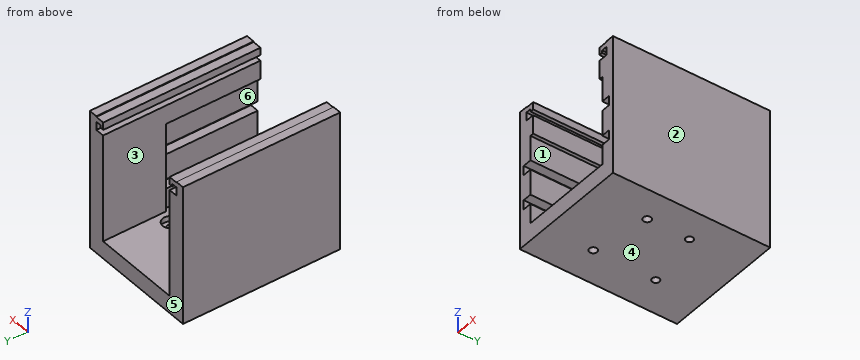
```python
from build123d import *

# Parameters (mm, degrees)
SKETCH1_W                                     = 90
SKETCH1_H                                     = 70
BOSS_EXTRUDE1_DEPTH                           = 10
SKETCH2_W                                     = 8
SKETCH2_H                                     = 90
BOSS_EXTRUDE2_DEPTH                           = 51
SKETCH3_W                                     = 5.1
SKETCH3_H                                     = 5.4
CUT_EXTRUDE1_DEPTH                            = 54
SKETCH14_W                                    = 10
SKETCH14_H                                    = 90
BOSS_EXTRUDE6_DEPTH                           = 11.75
SKETCH15_W                                    = 4.9
SKETCH15_H                                    = 90
BOSS_EXTRUDE7_DEPTH                           = 7
SKETCH17_W                                    = 90
SKETCH17_H                                    = 2.8
BOSS_EXTRUDE8_DEPTH                           = 5
SKETCH16_W                                    = 5.1
SKETCH16_H                                    = 90
CUT_EXTRUDE3_DEPTH                            = 1
BOSS_EXTRUDE9_START                           = -1.5
SKETCH18_W                                    = 2
SKETCH18_H                                    = 90
BOSS_EXTRUDE9_DEPTH                           = 4.3
SKETCH43_W                                    = 36
SKETCH43_H                                    = 51
BOSS_EXTRUDE10_DEPTH                          = 2
SKETCH21_R                                    = 2.1
CUT_EXTRUDE7_DEPTH                            = 99.030926243
CBORE_FOR_M4_PAN_HEAD_MACHINE_SCREW4_AT_COUNT = 2
CBORE_FOR_M4_PAN_HEAD_MACHINE_SCREW4_AT_PITCH = 33.407334524
ADVANCEDHOLE1_START                           = 6.9
ADVANCEDHOLE1_OUTLINE_R                       = 4.5
ADVANCEDHOLE1_OUTLINE_R_2                     = 2.1
ADVANCEDHOLE1_DEPTH                           = 3.1


# Read off the part's stored shape, not the designer's step: AdvancedHole1
with BuildPart() as part:
    # Sketch1 → Boss-Extrude1 (new body)
    with BuildSketch(Plane(origin=(0, 0, 0), x_dir=(0, 1, 0), z_dir=(0, 0, 1))):
        Rectangle(SKETCH1_W, SKETCH1_H)
    extrude(amount=BOSS_EXTRUDE1_DEPTH)

    # Sketch2 → Boss-Extrude2 (add)
    with BuildSketch(Plane.XY.offset(10)):
        with Locations((-31, 0)):
            Rectangle(SKETCH2_W, SKETCH2_H)
        with Locations((31, 0)):
            Rectangle(SKETCH2_W, SKETCH2_H)
    extrude(amount=BOSS_EXTRUDE2_DEPTH)

    # Sketch3 → Cut-Extrude1 (cut)
    with BuildSketch(Plane.XZ.offset(45)):
        with Locations((-29.55, 24)):
            Rectangle(SKETCH3_W, SKETCH3_H)
        with Locations((-29.55, 44)):
            Rectangle(SKETCH3_W, SKETCH3_H)
        with Locations((29.55, 24)):
            Rectangle(SKETCH3_W, SKETCH3_H)
        with Locations((29.55, 44)):
            Rectangle(SKETCH3_W, SKETCH3_H)
    extrude(amount=-CUT_EXTRUDE1_DEPTH, mode=Mode.SUBTRACT)

    # Sketch14 → Boss-Extrude6 (add)
    with BuildSketch(Plane.XY.offset(61)):
        with Locations((30, 0)):
            Rectangle(SKETCH14_W, SKETCH14_H)
    boss_extrude6 = extrude(amount=BOSS_EXTRUDE6_DEPTH)

    # Sketch15 → Boss-Extrude7 (add)
    with BuildSketch(Plane.XY.offset(72.75)):
        with Locations((32.55, 0)):
            Rectangle(SKETCH15_W, SKETCH15_H)
    boss_extrude7 = extrude(amount=BOSS_EXTRUDE7_DEPTH)

    # Sketch17 → Boss-Extrude8 (add)
    with BuildSketch(Plane(origin=(30.1, 0, 0), x_dir=(0, -1, 0), z_dir=(-1, 0, 0))):
        with Locations((0, 77.95)):
            Rectangle(SKETCH17_W, SKETCH17_H)
    boss_extrude8 = extrude(amount=BOSS_EXTRUDE8_DEPTH)

    # Sketch16 → Cut-Extrude3 (cut)
    with BuildSketch(Plane.XY.offset(72.75)):
        with Locations((27.55, 0)):
            Rectangle(SKETCH16_W, SKETCH16_H)
    cut_extrude3 = extrude(amount=-CUT_EXTRUDE3_DEPTH, mode=Mode.SUBTRACT)

    # Sketch18 → Boss-Extrude9 (add)
    with BuildSketch(Plane.XY.offset(76.55).offset(BOSS_EXTRUDE9_START)):
        with Locations((25.9, 0)):
            Rectangle(SKETCH18_W, SKETCH18_H)
    boss_extrude9 = extrude(amount=BOSS_EXTRUDE9_DEPTH)

    # Sketch43 → Boss-Extrude10 (add)
    with BuildSketch(Plane(origin=(27, 0, 0), x_dir=(0, -1, 0), z_dir=(-1, 0, 0))):
        with Locations((-27, 35.5)):
            Rectangle(SKETCH43_W, SKETCH43_H)
    boss_extrude10 = extrude(amount=BOSS_EXTRUDE10_DEPTH)

    # Mirror2: Boss-Extrude6, Boss-Extrude7, Boss-Extrude8, Cut-Extrude3, Boss-Extrude9, Boss-Extrude10 across plane
    add(boss_extrude6.mirror(Plane(origin=(0, 0, 0), x_dir=(0, 0, 1), z_dir=(1, 0, 0))))
    add(boss_extrude7.mirror(Plane(origin=(0, 0, 0), x_dir=(0, 0, 1), z_dir=(1, 0, 0))))
    add(boss_extrude8.mirror(Plane(origin=(0, 0, 0), x_dir=(0, 0, 1), z_dir=(1, 0, 0))))
    add(cut_extrude3.mirror(Plane(origin=(0, 0, 0), x_dir=(0, 0, 1), z_dir=(1, 0, 0))), mode=Mode.SUBTRACT)
    add(boss_extrude9.mirror(Plane(origin=(0, 0, 0), x_dir=(0, 0, 1), z_dir=(1, 0, 0))))
    add(boss_extrude10.mirror(Plane(origin=(0, 0, 0), x_dir=(0, 0, 1), z_dir=(1, 0, 0))))

    # Sketch21 → Cut-Extrude7 (cut, through all)
    with BuildSketch(Plane(origin=(0, 0, 0), x_dir=(1, 0, 0), z_dir=(0, 0, -1))):
        with Locations((17.5, 12.1)):
            Circle(SKETCH21_R)
        with Locations(Location((17.5, -12.1, 0), (0, 0, 180))):
            Circle(SKETCH21_R)
        with Locations(Location((-15.4, -17.9, 0), (0, 0, 180))):
            Circle(SKETCH21_R)
        with Locations((-15.4, 17.9)):
            Circle(SKETCH21_R)
    extrude(amount=-CUT_EXTRUDE7_DEPTH, mode=Mode.SUBTRACT)

    # Sketch30 → CBORE for M4 Pan Head Machine Screw4 (revolve, cut)
    with BuildSketch(Plane(origin=(17.5, -12.1, 10), x_dir=(0, -1, 0), z_dir=(1, 0, 0))):
        Polygon((0, 0), (0, 10), (2.25, 10), (2.25, 3.1), (4.5, 3.1), (4.5, 0.025), (4.525, 0), align=None)
    cbore_for_m4_pan_head_machine_screw4 = revolve(axis=Axis((17.5, -12.1, 16.35), (0, 0, -1)), mode=Mode.SUBTRACT)

    # CBORE for M4 Pan Head Machine Screw4 at: CBORE for M4 Pan Head Machine Screw4 ×2
    with Locations(*[Vector(-0.9848136784555953, -0.1736145694541778, 0) * (i * CBORE_FOR_M4_PAN_HEAD_MACHINE_SCREW4_AT_PITCH) for i in range(1, CBORE_FOR_M4_PAN_HEAD_MACHINE_SCREW4_AT_COUNT)]):
        add(cbore_for_m4_pan_head_machine_screw4, mode=Mode.SUBTRACT)

    # AdvancedHole1 outline → AdvancedHole1 (cut)
    # profile 1 of 2: a face of its own
    with BuildSketch(Plane.XY.offset(ADVANCEDHOLE1_START)):
        with Locations((17.5, 12.1)):
            Circle(ADVANCEDHOLE1_OUTLINE_R)
        with Locations((17.5, 12.1)):
            Circle(ADVANCEDHOLE1_OUTLINE_R_2, mode=Mode.SUBTRACT)
    # profile 2 of 2: a face of its own
    with BuildSketch(Plane.XY.offset(ADVANCEDHOLE1_START)):
        with Locations((-15.4, 17.9)):
            Circle(ADVANCEDHOLE1_OUTLINE_R)
        with Locations((-15.4, 17.9)):
            Circle(ADVANCEDHOLE1_OUTLINE_R_2, mode=Mode.SUBTRACT)
    extrude(amount=ADVANCEDHOLE1_DEPTH, mode=Mode.SUBTRACT)


solid = part.part
```
The listing builds one solid part. Answer for the finished solid, in the listing's coordinates (mm). Face numbers are marked on the shaded views. A direction names the side the tool comes from. Round coordinates to 2 decimals unless told otherwise and drop trailing zeros. Loops run counter-clockwise (first coordinate to the right, second up) from the corner with the lowest first, then second, coordinate; pieces in that order, holes last.
Q1. For a pull along Z with two mould halves and no side action, classify the marked faces 4, 5 and 6 as released by +Z, released by -Z, zero draft, split by the parting line, or undercut.
Q2. Section B-B, the plane z = 37.5 is taken. Determine the outline of the cut face in (x, y).
Q3. Section A-A, the plane x = -15.4 is taken. Determine the outline of the cut face in (y, z) (3 decimals).
Q4. Which of the six approach directions +Z, -Z, +X, -X, +Y, -Y give full straight-line access (tool end or side, diameter ignored) to the marked faces 1, 2 and 3?
Q5. Find the intervals of material crossed by line 1 (Y direction, x = 17.5, z = 8.6); line 2 (X direction, y = -15.5, z = 33.5); line 3 (Y direction, x = -15, z = 4), in increasing order.
Q6. Given pin 1 Ø7 at (x, y) = (18.5, -10.5) entering from +Z; pin 2 Ø4 at (x, y) = (-27.5, 11.5) entering from +Z, each flat-ended and moving along its own axis, determine where each tip first touches the part or whether it passes through.
Q7. Section D-D, the plane y = 39.5 is taken. Determine the outline of the cut face in (x, z), then the cut area to 3 significant figures.
Completed:
1. face 4: released by -Z
1. face 5: zero draft
1. face 6: undercut
2. outline: (-35, -45) - (-27, -45) - (-27, 9) - (-25, 9) - (-25, 45) - (-35, 45) - close; (25, 9) - (27, 9) - (27, -45) - (35, -45) - (35, 45) - (25, 45) - close
3. outline: (-45, 0) - (-20.15, 0) - (-20.15, 6.9) - (-22.4, 6.9) - (-22.4, 9.975) - (-22.425, 10) - (-45, 10) - close; (-15.65, 0) - (15.8, 0) - (15.8, 6.9) - (13.4, 6.9) - (13.4, 10) - (-13.375, 10) - (-13.4, 9.975) - (-13.4, 6.9) - (-15.65, 6.9) - close; (20, 0) - (45, 0) - (45, 10) - (22.4, 10) - (22.4, 6.9) - (20, 6.9) - close
4. face 1: -Y
4. face 2: +Z, -Z, +X, +Y, -Y
4. face 3: +Y, -Y
5. line 1: y = -45 to -16.6, -7.6 to 7.6, 16.6 to 45
5. line 2: x = -35 to -27, 27 to 35
5. line 3: y = -45 to -20.11, -15.69 to 15.84, 19.96 to 45
6. pin 1: stops at z = 10
6. pin 2: stops at z = 79.35
7. outline: (-35, 0) - (35, 0) - (35, 79.75) - (30.1, 79.75) - (30.1, 79.35) - (24.9, 79.35) - (24.9, 75.05) - (26.9, 75.05) - (26.9, 76.55) - (30.1, 76.55) - (30.1, 71.75) - (25, 71.75) - (25, 10) - (-25, 10) - (-25, 71.75) - (-30.1, 71.75) - (-30.1, 76.55) - (-26.9, 76.55) - (-26.9, 75.05) - (-24.9, 75.05) - (-24.9, 79.35) - (-30.1, 79.35) - (-30.1, 79.75) - (-35, 79.75) - close
7. area: 2,050 mm2
